Input: part model. Units: mm. Frame: model coordinates. Face numbers are marked on the shaded views. Coordinates: 2 decimals unless noted, no trailing zeros. Loops run counter-clockwise (first coordinate to the right, second up) from the corner with the lowest first, then second, coordinate; pieces in that order, holes last. Notation, with made-up numbers: (-13, -29) - (46, -29) arc R34 cw to (46, 10) - close; hole circle Ø9 at (16.25, 55). An arc over 180 degrees is marked (long way). Answer as CSV lines item,"result". Start each with the question number.
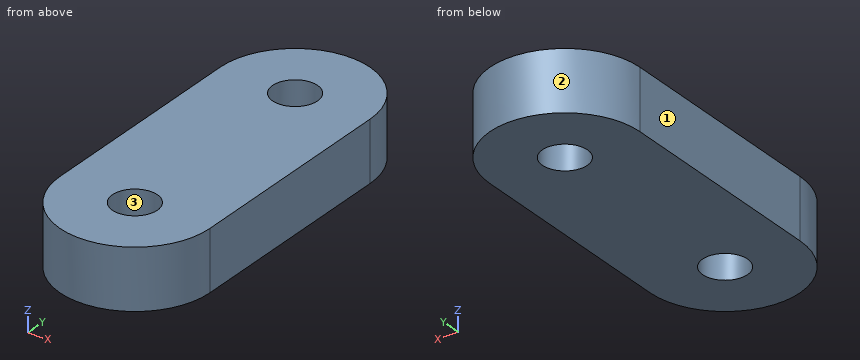
```python
from build123d import *

# Parameters (mm, degrees)
F0_R     = 1.5
F1_DEPTH = 4


with BuildPart() as f1:
    # F0 (on Top) → F1 (new body)
    with BuildSketch(Plane.XY):
        with BuildLine():
            ThreePointArc((-5, 6.816642), (0, 1.816642), (5, 6.816642))
            ThreePointArc((5, 6.816642), (0, 11.816642), (-5, 6.816642))
        make_face()
        with Locations((0, 6.816642)):
            Circle(F0_R, mode=Mode.SUBTRACT)
        with BuildLine():
            Line((5, -8.183358), (5, 6.816642))
            ThreePointArc((5, 6.816642), (0, 1.816642), (-5, 6.816642))
            Line((-5, 6.816642), (-5, -8.183358))
            ThreePointArc((-5, -8.183358), (0, -3.183358), (5, -8.183358))
        make_face()
        with BuildLine():
            ThreePointArc((-5, -8.183358), (0, -13.183358), (5, -8.183358))
            ThreePointArc((5, -8.183358), (0, -3.183358), (-5, -8.183358))
        make_face()
        with Locations((0, -8.183358)):
            Circle(F0_R, mode=Mode.SUBTRACT)
    extrude(amount=F1_DEPTH)


solid = f1.part
```
Item 1: Contact query for a flat-ended pin moving along its axis: P1, Ø2.5, axis at x = 0, y = -8.18, coming from the +Z side. Output: stop coordinate, or through.
Item 2: Section query C-C, the plane z = 2.6. Output: boundary loops of the cut face in (x, y), and give its area (3 significant figures).
Item 3: Section query B-B, the plane y = -7.75. Output: boundary loops of the cut face in (x, z).
Item 4: Draft query along Y for the marked faces 1, 2 and 3. Return one class per face: pulls with the +Y half, pulls with the -Y half, needs draft (parallel to the pull), parting line crosses it, or undercut.
Item 5: Material intervals for probe 1 along Y at (x, z) = (0, 2.3); probe 2 along X at (y, z) = (-8, 0.35); probe 3 along Y at (x, z) = (1.25, 1.15), sorted ascending.
Item 6: Section query D-D, the plane x = 4.25. Output: boundary loops of the cut face in (y, z), and give its area (3 significant figures).
Item 7: Section query A-A, the plane x = 0. Output: boundary loops of the cut face in (y, z).
Response values:
1,P1,"passes through"
2,outline,"(-5, -8.18) arc R5 ccw to (5, -8.18) - (5, 6.82) arc R5 ccw to (-5, 6.82) - close; hole circle Ø3 at (0, -8.18); hole circle Ø3 at (0, 6.82)"
2,area,"214 mm²"
3,outline,"(-5, 0) - (-1.44, 0) - (-1.44, 4) - (-5, 4) - close; (1.44, 0) - (5, 0) - (5, 4) - (1.44, 4) - close"
4,face 1,"needs draft"
4,face 2,"pulls with the +Y half"
4,face 3,"undercut"
5,probe 1,"y = -13.18 to -9.68, -6.68 to 5.32, 8.32 to 11.82"
5,probe 2,"x = -5 to -1.49, 1.49 to 5"
5,probe 3,"y = -13.02 to -9.01, -7.35 to 5.99, 7.65 to 11.66"
6,outline,"(-10.82, 0) - (9.45, 0) - (9.45, 4) - (-10.82, 4) - close"
6,area,"81.1 mm²"
7,outline,"(-13.18, 0) - (-9.68, 0) - (-9.68, 4) - (-13.18, 4) - close; (-6.68, 0) - (5.32, 0) - (5.32, 4) - (-6.68, 4) - close; (8.32, 0) - (11.82, 0) - (11.82, 4) - (8.32, 4) - close"
